from build123d import *

# Parameters (mm, degrees)
BOSS_EXTRUDE1_DEPTH                                 = 9.525
SKETCH4_W                                           = 50.8
SKETCH4_H                                           = 200
BOSS_EXTRUDE2_DEPTH                                 = 9.525
CSK_FOR_1_4_FLAT_HEAD_MACHINE_SCREW_100_D           = 6.7564
CSK_FOR_1_4_FLAT_HEAD_MACHINE_SCREW_100_CSINK_D     = 17.6447958
CSK_FOR_1_4_FLAT_HEAD_MACHINE_SCREW_100_CSINK_ANGLE = 100
LPATTERN1_COUNT                                     = 2
LPATTERN1_PITCH                                     = 491.2
LPATTERN1_COUNT_DIR2                                = 5
LPATTERN1_PITCH_DIR2                                = 287.65
LPATTERN2_COUNT                                     = 3
LPATTERN2_PITCH                                     = 163.733333333
LPATTERN2_COUNT_DIR2                                = 2
LPATTERN2_PITCH_DIR2                                = 76.2
CSK_FOR_1_4_FLAT_HEAD_MACHINE_SCREW_2_D             = 6.7564
CSK_FOR_1_4_FLAT_HEAD_MACHINE_SCREW_2_CSINK_D       = 17.6447958
CSK_FOR_1_4_FLAT_HEAD_MACHINE_SCREW_2_CSINK_ANGLE   = 100
FILLET1_R                                           = 3.175
FILLET2_R                                           = 3.175


with BuildPart() as part:
    # Sketch1 → Boss-Extrude1 (new body)
    with BuildSketch(Plane(origin=(0, 0, 0), x_dir=(1, 0, 0), z_dir=(0, 1, 0))):
        Polygon((-258.3, 0), (-207.5, 0), (-207.5, 1074.4), (207.5, 1074.4), (207.5, 0), (258.3, 0), (258.3, 1113.914856628), (230.3, 1117.85), (-61.7, 1117.85), (-61.7, 1132.55), (271.3, 1132.55), (271.3, 1176), (-258.3, 1176), align=None)
    extrude(amount=BOSS_EXTRUDE1_DEPTH)

    # Sketch4 → Boss-Extrude2 (add)
    with BuildSketch(Plane.XZ):
        with Locations((-232.9, -1276)):
            Rectangle(SKETCH4_W, SKETCH4_H)
        with Locations((232.9, -1276)):
            Rectangle(SKETCH4_W, SKETCH4_H)
    extrude(amount=-BOSS_EXTRUDE2_DEPTH)

    # CSK for 1_4 Flat Head Machine Screw _100 (through all)
    with Locations(Plane.XZ):
        with Locations((-245.6, -1163.3)):
            csk_for_1_4_flat_head_machine_screw_100 = CounterSinkHole(CSK_FOR_1_4_FLAT_HEAD_MACHINE_SCREW_100_D / 2, CSK_FOR_1_4_FLAT_HEAD_MACHINE_SCREW_100_CSINK_D / 2, counter_sink_angle=CSK_FOR_1_4_FLAT_HEAD_MACHINE_SCREW_100_CSINK_ANGLE)

    # LPattern1: CSK for 1_4 Flat Head Machine Screw _100 2 × 5
    with Locations(*[(i * LPATTERN1_PITCH, 0, j * LPATTERN1_PITCH_DIR2) for i in range(LPATTERN1_COUNT) for j in range(LPATTERN1_COUNT_DIR2) if (i, j) != (0, 0)]):
        add(csk_for_1_4_flat_head_machine_screw_100, mode=Mode.SUBTRACT)

    # LPattern2: CSK for 1_4 Flat Head Machine Screw _100 3 × 2, 1 skipped
    with Locations(*[(i * LPATTERN2_PITCH, 0, j * LPATTERN2_PITCH_DIR2) for i in range(LPATTERN2_COUNT) for j in range(LPATTERN2_COUNT_DIR2) if (i, j) not in ((0, 0), (0, 1))]):
        add(csk_for_1_4_flat_head_machine_screw_100, mode=Mode.SUBTRACT)

    # CSK for 1_4 Flat Head Machine Screw  2 (through all)
    with Locations(Plane.XZ):
        with Locations((-245.6, -1363.3)):
            csk_for_1_4_flat_head_machine_screw_2 = CounterSinkHole(CSK_FOR_1_4_FLAT_HEAD_MACHINE_SCREW_2_D / 2, CSK_FOR_1_4_FLAT_HEAD_MACHINE_SCREW_2_CSINK_D / 2, counter_sink_angle=CSK_FOR_1_4_FLAT_HEAD_MACHINE_SCREW_2_CSINK_ANGLE)

    # Mirror1: CSK for 1_4 Flat Head Machine Screw  2 across plane
    add(csk_for_1_4_flat_head_machine_screw_2.mirror(Plane(origin=(0, 0, 0), x_dir=(0, 0, 1), z_dir=(1, 0, 0))), mode=Mode.SUBTRACT)

    # Fillet1
    fillet1_edges = [part.edges().sort_by_distance(p)[0] for p in [
        (258.3, 4.7625, 0),
        (207.5, 4.7625, 0),
        (-207.5, 4.7625, 0),
        (-258.3, 4.7625, 0),
        (207.5, 4.7625, -1074.4),
        (-207.5, 4.7625, -1074.4),
        (258.3, 4.7625, -1113.914856628),
        (271.3, 4.7625, -1132.55),
        (271.3, 4.7625, -1176),
        (-61.7, 4.7625, -1117.85),
        (-61.7, 4.7625, -1132.55),
    ]]
    fillet(fillet1_edges, radius=FILLET1_R)

    # Fillet2
    fillet2_edges = [part.edges().sort_by_distance(p)[0] for p in [
        (207.5, 4.7625, -1376),
        (258.3, 4.7625, -1376),
        (-258.3, 4.7625, -1376),
        (-207.5, 4.7625, -1376),
        (-207.5, 4.7625, -1176),
        (207.5, 4.7625, -1176),
        (258.3, 4.7625, -1176),
    ]]
    fillet(fillet2_edges, radius=FILLET2_R)


solid = part.part
The listing builds one solid part. Answer for the finished solid, in the listing's coordinates (mm). Give positions to 0.01 mm unless a question says otherwise; leave off trailing zeros. Order: outer loops, then holes, each group sorted by start corner. A loop starts at its lowest first (then second) coordinate and runs counter-clockwise, first axis right, second up. Notation, with made-up numbers: (5.5, -0.75) - (17.5, -0.75) arc R21 ccw to (17.5, 5.25) - close; hole circle Ø4 at (33.5, 36.25). An arc over 180 degrees is marked (long way). Use one line per item in the form item = value.
1) Find section B-B on x = -167. Determine the outline of the cut face in (y, z) (3 decimals).
Verdict:
outline = (0, -1176) - (9.525, -1176) - (9.525, -1074.4) - (0, -1074.4) - close
2) Find section A-A on z = -1258. Determine the outline of the cut face in (x, y) (3 decimals), and give its area (3 significant figures).
Verdict:
outline = (-258.3, 0) - (-207.5, 0) - (-207.5, 9.525) - (-258.3, 9.525) - close; (207.5, 0) - (258.3, 0) - (258.3, 9.525) - (207.5, 9.525) - close
area = 968 mm^2
3) Each of these flat-tipped pins is pushed along its axis until it touches: pin 1 (5.5 mm diameter, centred on x = -245.6, z = -875.65, fed in from -Y); pin 2 (1 mm diameter, centred on y = 3.5, z = -1072.5, fed in from +X); pin 3 (11 mm diameter, centred on x = -245.6, z = -588, fed in from -Y); pin 4 (3 mm diameter, centred on x = 98, y = 2.5, fed in from -Z). Where does it stop, or does it pass through?
Verdict:
pin_1 = through
pin_2 = 258.3
pin_3 = 2.79
pin_4 = -1176
4) Consider probe 1 along X at (y, z) = (6.6, -1087.1); probe 2 along X at (y, z) = (8.35, -300.35); probe 3 along X at (y, z) = (7.25, -1164). Determine where each line is inside the solid, lowest interval first. Write a range as [from, to].
Verdict:
probe_1 = [-258.3, -85.24], [-78.49, 78.49], [85.24, 258.3]
probe_2 = [-258.3, -248.98], [-242.22, -207.5], [207.5, 242.22], [248.98, 258.3]
probe_3 = [-258.3, -248.9], [-242.3, -85.17], [-78.56, 78.56], [85.17, 242.3], [248.9, 271.3]
